```python
from build123d import *

# Parameters (mm, degrees)
SKETCH1_R           = 44.45
BOSS_EXTRUDE1_DEPTH = 5
SKETCH2_R           = 38.1
BOSS_EXTRUDE2_DEPTH = 10
SKETCH3_R           = 44.45
BOSS_EXTRUDE3_DEPTH = 5
BOSS_EXTRUDE4_DEPTH = 5
SKETCH5_R           = 13.5
BOSS_EXTRUDE5_DEPTH = 15
SKETCH6_R           = 13.5
BOSS_EXTRUDE6_DEPTH = 15
SKETCH7_R           = 11
CUT_EXTRUDE1_DEPTH  = 14
SKETCH8_R           = 11
CUT_EXTRUDE2_DEPTH  = 14


with BuildPart() as part:
    # Sketch1 → Boss-Extrude1 (new body)
    with BuildSketch(Plane(origin=(0, 0, 0), x_dir=(1, 0, 0), z_dir=(0, 1, 0))):
        Circle(SKETCH1_R)
    extrude(amount=BOSS_EXTRUDE1_DEPTH)

    # Sketch2 → Boss-Extrude2 (add)
    with BuildSketch(Plane(origin=(0, 5, 0), x_dir=(1, 0, 0), z_dir=(0, 1, 0))):
        Circle(SKETCH2_R)
    extrude(amount=BOSS_EXTRUDE2_DEPTH)

    # Sketch3 → Boss-Extrude3 (add)
    with BuildSketch(Plane(origin=(0, 15, 0), x_dir=(1, 0, 0), z_dir=(0, 1, 0))):
        Circle(SKETCH3_R)
    extrude(amount=BOSS_EXTRUDE3_DEPTH)

    # Sketch4 → Boss-Extrude4 (add)
    with BuildSketch(Plane(origin=(0, 0, 0), x_dir=(1, 0, 0), z_dir=(0, 1, 0))):
        with BuildLine():
            ThreePointArc((-44.195335285, -4.751298672), (-44.443598423, -0.75436016), (-44.331122698, 3.248701328))
            Line((-44.331122698, 3.248701328), (-73.805449313, 3.248701328))
            Line((-73.805449313, 3.248701328), (-73.805449313, -4.751298672))
            Line((-73.805449313, -4.751298672), (-44.195335285, -4.751298672))
        make_face()
        with BuildLine():
            Line((73.805449313, 3.248701328), (44.331122698, 3.248701328))
            ThreePointArc((44.331122698, 3.248701328), (44.420270733, 1.625437797), (44.45, 0))
            ThreePointArc((44.45, 0), (44.386288161, -2.37905933), (44.195335285, -4.751298672))
            Line((44.195335285, -4.751298672), (73.805449313, -4.751298672))
            Line((73.805449313, -4.751298672), (73.805449313, 3.248701328))
        make_face()
    extrude(amount=BOSS_EXTRUDE4_DEPTH)

    # Sketch5 → Boss-Extrude5 (add)
    with BuildSketch(Plane.ZY.offset(73.805449313)):
        with Locations((0.751298672, 5)):
            Circle(SKETCH5_R)
    extrude(amount=BOSS_EXTRUDE5_DEPTH)

    # Sketch6 → Boss-Extrude6 (add)
    with BuildSketch(Plane(origin=(73.805449313, 0, 0), x_dir=(0, 0, -1), z_dir=(1, 0, 0))):
        with Locations((-0.751298672, 5)):
            Circle(SKETCH6_R)
    extrude(amount=BOSS_EXTRUDE6_DEPTH)

    # Sketch7 → Cut-Extrude1 (cut)
    with BuildSketch(Plane(origin=(88.805449313, 0, 0), x_dir=(0, 0, -1), z_dir=(1, 0, 0))):
        with Locations((-0.751298672, 5)):
            Circle(SKETCH7_R)
    extrude(amount=-CUT_EXTRUDE1_DEPTH, mode=Mode.SUBTRACT)

    # Sketch8 → Cut-Extrude2 (cut)
    with BuildSketch(Plane.ZY.offset(88.805449313)):
        with Locations((0.751298672, 5)):
            Circle(SKETCH8_R)
    extrude(amount=-CUT_EXTRUDE2_DEPTH, mode=Mode.SUBTRACT)


solid = part.part
```
CAD build for the part. Positions are in the model's coordinates, mm. A direction names the side the tool comes from. Round coordinates to 2 decimals unless told otherwise and drop trailing zeros. Order: outer loops, then holes, each group sorted by start corner. A loop starts at its lowest first (then second) coordinate and runs counter-clockwise, first axis right, second up.
Q1. Drop flat-ended pins along their axis: pin 1 (4 mm diameter, centred on y = 10, z = -23, fed in from -X); pin 2 (6 mm diameter, centred on x = 4.5, y = 13, fed in from +Z); pin 3 (1.5 mm diameter, centred on x = 54.5, y = 1.5, fed in from -Z). Give the stop position or say it passes through.
Q2. Slice it at D-D (z = 0). Write the cut outline in (x, y).
Q3. Slice it at A-A (z = -28). Write the cut outline in (x, y).
Q4. Slice it at C-C (x = 18). Write the cut outline in (y, z), and give its area (3 significant figures).
Q5. Wall check: L1, parallel to X at y = 5.75, z = 12.5; L2, parallel to Y at x = 17.5, z = 35; L3, parallel to X at y = -6.5, z = 0.5. Give the ranges that are in metal, low to high.
Q6. Slice it at B-B (x = 60.5). Write the cut outline in (y, z), and give its area (3 significant figures).
Q7. Two-plate mould, pull along Y, no slides. Class faces 1 (the cylindrical face through (-81.2, 5.594, -12.736)), 2 (the flat face through (-74.805, 5, 1)), 3 (the flat face through (-1, 20, -1)), 4 (the flat face through (-73.805, 5.2, 0.6)): pulls with the +Y half, pulls with the -Y half, needs draft (parallel to the pull), parting line crosses it, or undercut.
Q8. Which spindle directions (+Z, -Z, +X, -X, +Y, -Y) get a long thin tool onto all of the face, cutting with end or side? Do faces 5 (the flat face through (-1, 0, -1)), 6 (the flat face through (59, 2, 4.751)), 7 (the flat face through (-33, 5, 20)), 8 (the cylindrical face through (81.903, -5.738, 3.136)), 9 (the cylindrical face through (-81.9, 5.48, -10.24)). Say none if no direction does.
Results below:
1. pin 1: stops at x = -31.79
1. pin 2: stops at z = 44.39
1. pin 3: stops at z = -3.25
2. outline: (-88.81, -8.48) - (-73.81, -8.48) - (-73.81, 0) - (73.81, 0) - (73.81, -8.48) - (88.81, -8.48) - (88.81, -5.97) - (74.81, -5.97) - (74.81, 15.97) - (88.81, 15.97) - (88.81, 18.48) - (73.81, 18.48) - (73.81, 5) - (38.1, 5) - (38.1, 15) - (44.45, 15) - (44.45, 20) - (-44.45, 20) - (-44.45, 15) - (-38.1, 15) - (-38.1, 5) - (-73.81, 5) - (-73.81, 18.48) - (-88.81, 18.48) - (-88.81, 15.97) - (-74.81, 15.97) - (-74.81, -5.97) - (-88.81, -5.97) - close
3. outline: (-34.52, 0) - (34.52, 0) - (34.52, 5) - (25.84, 5) - (25.84, 15) - (34.52, 15) - (34.52, 20) - (-34.52, 20) - (-34.52, 15) - (-25.84, 15) - (-25.84, 5) - (-34.52, 5) - close
4. outline: (0, -40.64) - (5, -40.64) - (5, -33.58) - (15, -33.58) - (15, -40.64) - (20, -40.64) - (20, 40.64) - (15, 40.64) - (15, 33.58) - (5, 33.58) - (5, 40.64) - (0, 40.64) - close
4. area: 1,480 mm2
5. L1: x = -88.81 to -73.81, -35.99 to 35.99, 73.81 to 88.81
5. L2: y = 0 to 5, 15 to 20
5. L3: x = -88.81 to -73.81, 73.81 to 88.81
6. outline: (0, -3.25) - (5, -3.25) - (5, 4.75) - (0, 4.75) - close
6. area: 40.0 mm2
7. face 1: parting line crosses it
7. face 2: undercut
7. face 3: pulls with the +Y half
7. face 4: needs draft
8. face 5: +Z, -Z, -Y
8. face 6: +Z, +Y, -Y
8. face 7: none
8. face 8: +X
8. face 9: -X
